The listing builds one solid part. Answer for the finished solid, in the listing's coordinates (mm). Round coordinates to 2 decimals unless told otherwise and drop trailing zeros. Order: outer loops, then holes, each group sorted by start corner. A loop starts at its lowest first (then second) coordinate and runs counter-clockwise, first axis right, second up. Notation, with made-up numbers: (58, 71.25) - (62, 71.25) arc R30 cw to (62, 98.25) - close; hole circle Ø11 at (82, 84). An arc over 180 degrees is marked (long way). One line per item, written item: value. Start each with the question number.
1. Straight lines are drawn through the part: line 1 (Z direction, x = -14.5, y = -12); line 2 (Z direction, x = -5.25, y = 14.5); line 3 (Y direction, x = -21, z = 41.5). For each, find the intervals that lie inside material, in ascending order.
2. Flat-ended cylindrical pins translate along their axes: P1, Ø8, axis at x = -22, y = 121, coming from the -Z side; P2, Ø1.5, axis at x = -19, y = 110, coming from the +Z side; P3, Ø5, axis at x = -4.5, z = -1.5, coming from the +Y side. Find the tip coordinate at first contact, or state that the pin passes through.
3. Section B-B, the plane y = -27.5 is taken. Give the vertices of the cut face in (x, z), then the cut area to 3 significant figures.
4. Section C-C, the plane z = 29 is taken. Give the vertices of the cut face in (x, y), then the cut area to 3 significant figures.
from build123d import *

# Parameters (mm, degrees)
F0_W     = 81.358406
F0_H     = 78.619389
F1_DEPTH = 25


with BuildPart() as f1:
    # F0 (on Right) → F1 (new body)
    with BuildSketch(Plane.YZ):
        Polygon((23.111533, -28.777307), (-58.246873, -28.777307), (35.977684, -75.584203), (147.975132, -57.679411), align=None)
        Polygon((147.975132, -57.679411), (23.111533, 49.842082), (23.111533, -28.777307), align=None)
        with Locations((-17.56767, 10.532387)):
            Rectangle(F0_W, F0_H)
    extrude(amount=-F1_DEPTH)


solid = f1.part
Answer list:
1. line 1: z = -51.75 to 49.84
1. line 2: z = -64.91 to 49.84
1. line 3: y = -58.25 to 32.8
2. P1: stops at z = -62.63
2. P2: stops at z = -24.33
2. P3: stops at y = 85.64
3. outline: (-25, -44.05) - (0, -44.05) - (0, 49.84) - (-25, 49.84) - close
3. area: 2,350 mm²
4. outline: (-25, -58.25) - (0, -58.25) - (0, 47.32) - (-25, 47.32) - close
4. area: 2,640 mm²
